Source: CAD feature listing. Evaluate the final solid. Frame: model axes, mm. A direction names the side the tool comes from. Round coordinates to 2 decimals unless told otherwise and drop trailing zeros. Write each loop counter-clockwise with the first axis right and the second up, starting at its lowest first coordinate (ties: lowest second). Pieces come first, ordered by that corner, then holes. Notation, with made-up numbers: M 66.5,-2 L 115.5,-2 A14 ccw 115.5,13 Z; hole C -2.5,25.25 d6. An arc over 180 degrees is marked long. Answer in a Markdown table with one row per item.
from build123d import *

# Parameters (mm, degrees)
SKETCH1_W             = 25.4
SKETCH1_H             = 5
BOSS_EXTRUDE1_DEPTH   = 6
SKETCH2_W             = 9
SKETCH2_H             = 0.79375
CUT_EXTRUDE1_DEPTH    = 27.218504915
SKETCH6_W             = 5
SKETCH6_H             = 6
BOSS_EXTRUDE2_DEPTH   = 6
F_8_CLEARANCE_HOLE1_D = 4.4958
FILLET1_R             = 2


with BuildPart() as part:
    # Sketch1 → Boss-Extrude1 (new body)
    with BuildSketch(Plane(origin=(0, 0, 0), x_dir=(1, 0, 0), z_dir=(0, 1, 0))):
        Rectangle(SKETCH1_W, SKETCH1_H)
    extrude(amount=BOSS_EXTRUDE1_DEPTH)

    # Sketch2 → Cut-Extrude1 (cut, through all)
    with BuildSketch(Plane(origin=(12.7, 0, 0), x_dir=(0, 0, -1), z_dir=(1, 0, 0))):
        with Locations((-2.5, 3)):
            Rectangle(SKETCH2_W, SKETCH2_H)
    extrude(amount=-CUT_EXTRUDE1_DEPTH, mode=Mode.SUBTRACT)

    # Sketch6 → Boss-Extrude2 (add)
    with BuildSketch(Plane(origin=(0, 0, -2.5), x_dir=(-1, 0, 0), z_dir=(0, 0, -1))):
        with Locations((10.2, 3)):
            Rectangle(SKETCH6_W, SKETCH6_H)
    extrude(amount=BOSS_EXTRUDE2_DEPTH)

    # #8 Clearance Hole1 (through all)
    with Locations(Plane(origin=(-7.7, 0, 0), x_dir=(0, 0, -1), z_dir=(1, 0, 0))):
        with Locations((5.5, 3)):
            Hole(F_8_CLEARANCE_HOLE1_D / 2)

    # Fillet1
    fillet1_edges = [part.edges().sort_by_distance(p)[0] for p in [
        (-10.2, 6, -8.5),
        (-10.2, 0, -8.5),
    ]]
    fillet(fillet1_edges, radius=FILLET1_R)

    # Mirror1: part across plane


with BuildPart() as part_1:
    add(part.part)
    add(part.part.mirror(Plane(origin=(0, 0, 0), x_dir=(0, 0, 1), z_dir=(1, 0, 0))))


solid = part_1.part
Q1. Pull-direction query (Z, two-part tool) for faces 1 (the cylindrical face through (-10.235, 3.099, -7.746)), 2 (the cylindrical face through (10.235, 3.099, -7.746)), 3 (the flat face through (-10, 3, -8.5)), 4 (the flat face through (0, 5, 2.5)); classes: pulls with the +Z half, pulls with the -Z half, needs draft (parallel to the pull), parting line crosses it, or undercut.
Solutions:
| item | result |
|---|---|
| face 1 | undercut |
| face 2 | undercut |
| face 3 | pulls with the -Z half |
| face 4 | pulls with the +Z half |
Q2. Material intervals for probe 1 along Y at (x, z) = (8.95, -5.5); probe 2 along X at (y, z) = (1.5, -3.25); probe 3 along Y at (x, z) = (9, 1), sorted ascending.
Solutions:
| item | result |
|---|---|
| probe 1 | y = 0 to 0.75, 5.25 to 6 |
| probe 2 | x = -12.7 to -7.7, 7.7 to 12.7 |
| probe 3 | y = 0 to 2.6, 3.4 to 6 |
Q3. Contact query for flat-ended pins moving along their axis: pin 1 Ø3 at (x, y) = (10, 5) entering from -Z; pin 2 Ø1 at (x, y) = (0.5, 4) entering from -Z. Output: stop coordinate, or through.
Solutions:
| item | result |
|---|---|
| pin 1 | stops at z = -8.5 |
| pin 2 | stops at z = -2.5 |
Q4. Section B-B (z = -1.5). Return loops of the section in (x, y).
Solutions:
| item | result |
|---|---|
| outline | M -12.7,0 L 12.7,0 L 12.7,2.6 L -12.7,2.6 Z; M -12.7,3.4 L 12.7,3.4 L 12.7,6 L -12.7,6 Z |
Q5. Section C-C (z = -5.5). Return loops of the section in (x, y).
Solutions:
| item | result |
|---|---|
| outline | M -12.7,0 L -7.7,0 L -7.7,0.75 L -12.7,0.75 Z; M -12.7,5.25 L -7.7,5.25 L -7.7,6 L -12.7,6 Z; M 7.7,0 L 12.7,0 L 12.7,0.75 L 7.7,0.75 Z; M 7.7,5.25 L 12.7,5.25 L 12.7,6 L 7.7,6 Z |
Q6. Section D-D (x = -9.75). Return loops of the section in (y, z).
Solutions:
| item | result |
|---|---|
| outline | M 0,-6.5 A2 ccw 2,-8.5 L 4,-8.5 A2 ccw 6,-6.5 L 6,2.5 L 3.4,2.5 L 3.4,-2 L 2.6,-2 L 2.6,2.5 L 0,2.5 Z; hole C 3,-5.5 d4.5 |
Q7. Section A-A (y = 3). Return loops of the section in (x, z), and give its area (3 significant figures).
Solutions:
| item | result |
|---|---|
| outline | M -12.7,-8.5 L -7.7,-8.5 L -7.7,-7.75 L -12.7,-7.75 Z; M -12.7,-3.25 L -7.7,-3.25 L -7.7,-2.5 L 7.7,-2.5 L 7.7,-3.25 L 12.7,-3.25 L 12.7,-2 L -12.7,-2 Z; M 7.7,-8.5 L 12.7,-8.5 L 12.7,-7.75 L 7.7,-7.75 Z |
| area | 27.7 mm2 |
Q8. Access query for faces 5 (the flat face through (-7.7, 4, -3)), 6 (the flat face through (0, 3.397, 0)), 7 (the cylindrical face through (10.24, 5.4, -7.93)). Directions: +Z, -Z, +X, -X, +Y, -Y. A direction counts if a zero-diameter tool reaches every point of the face in a straight line with its end or side. Return the directions, or none.
Solutions:
| item | result |
|---|---|
| face 5 | -Z, +Y, -Y |
| face 6 | +Z, +X, -X |
| face 7 | -Z, +X, -X, +Y |
